Read the model definition and answer for the solid it produces. Units are mm, in the model's axes. Coordinates: 2 decimals unless noted, no trailing zeros. Loops run counter-clockwise (first coordinate to the right, second up) from the corner with the lowest first, then second, coordinate; pieces in that order, holes last. Notation, with made-up numbers: M 45.5,58 L 79.5,58 A12 ccw 79.5,68 Z; hole C 88,77.25 d11. An arc over 180 degrees is marked long. One line per item, written item: value. Start each with the question number.
1. Flat-ended cylindrical pins translate along their axes: pin 1 (1.3 mm diameter, centred on x = 1.5, y = 51.5, fed in from +Z); pin 2 (1.3 mm diameter, centred on x = 1, z = -24.5, fed in from +Y); pin 3 (0.8 mm diameter, centred on x = 1.5, z = -24.5, fed in from -Y); pin 4 (1.5 mm diameter, centred on y = 17.5, z = -30, fed in from -X). Find the tip coordinate at first contact, or state that the pin passes through.
2. The part is cut by section B-B (y = -13). Write down the section's boundary in (x, z), then the cut area to 3 significant figures.
3. The part is cut by section C-C (z = 16). Write down the section's boundary in (x, y), then the cut area to 3 significant figures.
4. The part is cut by section A-A (x = 1.55). Write down the section's boundary in (y, z).
5. Consider probe 1 along Y at (x, z) = (0.8, -20.5); probe 2 along Z at (x, y) = (1, 57). Determine where each line is inside the solid, lowest interval first.
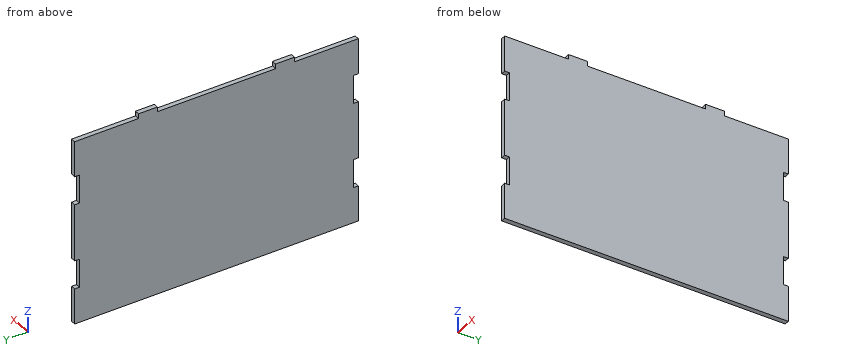
```python
from build123d import *

# Parameters (mm, degrees)
F0_W     = 152.4
F0_H     = 101.6
F1_DEPTH = 2.54
F2_W     = 34.29
F2_H     = 2.54
F2_W_2   = 63.5
F3_DEPTH = 25.4
F4_W     = 2.54
F4_H     = 15.24
F5_DEPTH = 25.4
F6_W     = 2.54
F6_H     = 15.24
F7_DEPTH = 25.4


with BuildPart() as f1:
    # F0 (on Right) → F1 (new body)
    with BuildSketch(Plane.YZ):
        Rectangle(F0_W, F0_H)
    extrude(amount=F1_DEPTH)

    # F2 (on face) → F3 (cut)
    with BuildSketch(Plane.YZ.offset(2.54)):
        with Locations((-59.055, 49.53)):
            Rectangle(F2_W, F2_H)
        with Locations((0, 49.53)):
            Rectangle(F2_W_2, F2_H)
        with Locations((59.055, 49.53)):
            Rectangle(F2_W, F2_H)
    extrude(amount=-F3_DEPTH, mode=Mode.SUBTRACT)

    # F4 (on face) → F5 (cut)
    with BuildSketch(Plane.YZ.offset(2.54)):
        with Locations((74.93, 21.59)):
            Rectangle(F4_W, F4_H)
        with Locations((74.93, -24.13)):
            Rectangle(F4_W, F4_H)
    extrude(amount=-F5_DEPTH, mode=Mode.SUBTRACT)

    # F6 (on face) → F7 (cut)
    with BuildSketch(Plane.YZ.offset(2.54)):
        with Locations((-74.93, 21.59)):
            Rectangle(F6_W, F6_H)
        with Locations((-74.93, -24.13)):
            Rectangle(F6_W, F6_H)
    extrude(amount=-F7_DEPTH, mode=Mode.SUBTRACT)


solid = f1.part
```
Answer block:
1. pin 1: stops at z = 48.26
1. pin 2: stops at y = 73.66
1. pin 3: stops at y = -73.66
1. pin 4: stops at x = 0
2. outline: M 0,-50.8 L 2.54,-50.8 L 2.54,48.26 L 0,48.26 Z
2. area: 252 mm2
3. outline: M 0,-73.66 L 2.54,-73.66 L 2.54,73.66 L 0,73.66 Z
3. area: 374 mm2
4. outline: M -76.2,-50.8 L 76.2,-50.8 L 76.2,-31.75 L 73.66,-31.75 L 73.66,-16.51 L 76.2,-16.51 L 76.2,13.97 L 73.66,13.97 L 73.66,29.21 L 76.2,29.21 L 76.2,48.26 L 41.91,48.26 L 41.91,50.8 L 31.75,50.8 L 31.75,48.26 L -31.75,48.26 L -31.75,50.8 L -41.91,50.8 L -41.91,48.26 L -76.2,48.26 L -76.2,29.21 L -73.66,29.21 L -73.66,13.97 L -76.2,13.97 L -76.2,-16.51 L -73.66,-16.51 L -73.66,-31.75 L -76.2,-31.75 Z
5. probe 1: y = -73.66 to 73.66
5. probe 2: z = -50.8 to 48.26
